```python
from build123d import *

# Parameters (mm, degrees)
SCHIZZO1_W                   = 27
SCHIZZO1_H                   = 20
SCHIZZO1_R                   = 1.4
ESTRUSIONE_ESTRUSIONE1_DEPTH = 2
RACCORDO1_R                  = 3
SCHIZZO2_R                   = 1.75
ESTRUSIONE_ESTRUSIONE2_DEPTH = 2.4
SCHIZZO3_R                   = 3
SCHIZZO3_R_2                 = 1.4
ESTRUSIONE_ESTRUSIONE3_DEPTH = 3


with BuildPart() as part:
    # Schizzo1 → Estrusione-Estrusione1 (new body)
    with BuildSketch(Plane.XY):
        Rectangle(SCHIZZO1_W, SCHIZZO1_H)
        with Locations((-10.5, 7)):
            Circle(SCHIZZO1_R, mode=Mode.SUBTRACT)
        with Locations((-10.5, -5.3)):
            Circle(SCHIZZO1_R, mode=Mode.SUBTRACT)
        with Locations((10.5, -5.3)):
            Circle(SCHIZZO1_R, mode=Mode.SUBTRACT)
        with Locations((10.5, 7)):
            Circle(SCHIZZO1_R, mode=Mode.SUBTRACT)
    extrude(amount=ESTRUSIONE_ESTRUSIONE1_DEPTH)

    # Raccordo1
    raccordo1_edges = [part.edges().sort_by_distance(p)[0] for p in [
        (-13.5, 10, 1),
        (13.5, 10, 1),
    ]]
    fillet(raccordo1_edges, radius=RACCORDO1_R)

    # Schizzo2 → Estrusione-Estrusione2 (add)
    with BuildSketch(Plane(origin=(13.5, 0, 0), x_dir=(0, 0, -1), z_dir=(1, 0, 0))):
        with BuildLine():
            Line((0, -10), (0, -14))
            ThreePointArc((0, -14), (-4.631989498, -17.094996434), (-5.718807717, -11.631192283))
            Line((-5.718807717, -11.631192283), (-2, -7.912384566))
            Line((-2, -7.912384566), (-2, -10))
            Line((-2, -10), (0, -10))
        make_face()
        with Locations((-3.35, -14)):
            Circle(SCHIZZO2_R, mode=Mode.SUBTRACT)
    estrusione_estrusione2 = extrude(amount=-ESTRUSIONE_ESTRUSIONE2_DEPTH)

    # Specchia1: Estrusione-Estrusione2 across plane
    add(estrusione_estrusione2.mirror(Plane(origin=(0, 0, 0), x_dir=(0, 0, 1), z_dir=(1, 0, 0))))

    # Schizzo3 → Estrusione-Estrusione3 (add)
    # profile 1 of 4: a face of its own
    with BuildSketch(Plane.XY.offset(2)):
        with Locations(Location((-10.5, 7, 0), (0, 0, 180))):
            Circle(SCHIZZO3_R)
        with Locations((-10.5, 7)):
            Circle(SCHIZZO3_R_2, mode=Mode.SUBTRACT)
    # profile 2 of 4: a face of its own
    with BuildSketch(Plane.XY.offset(2)):
        with Locations(Location((-10.5, -5.3, 0), (0, 0, 180))):
            Circle(SCHIZZO3_R)
        with Locations((-10.5, -5.3)):
            Circle(SCHIZZO3_R_2, mode=Mode.SUBTRACT)
    # profile 3 of 4: a face of its own
    with BuildSketch(Plane.XY.offset(2)):
        with Locations((10.5, -5.3)):
            Circle(SCHIZZO3_R)
        with Locations((10.5, -5.3)):
            Circle(SCHIZZO3_R_2, mode=Mode.SUBTRACT)
    # profile 4 of 4: a face of its own
    with BuildSketch(Plane.XY.offset(2)):
        with Locations((10.5, 7)):
            Circle(SCHIZZO3_R)
        with Locations((10.5, 7)):
            Circle(SCHIZZO3_R_2, mode=Mode.SUBTRACT)
    extrude(amount=ESTRUSIONE_ESTRUSIONE3_DEPTH)


solid = part.part
```
Model file for the job. Use its own axes, mm. A direction names the side the tool comes from. Coordinates: 2 decimals unless noted, no trailing zeros. Loops run counter-clockwise (first coordinate to the right, second up) from the corner with the lowest first, then second, coordinate; pieces in that order, holes last. Notation, with made-up numbers: M -8,-5 L 36,-5 A12 cw 36,0 Z; hole C 49.25,51 d3. An arc over 180 degrees is marked long. Use CSV: the item, a comma, the result in double quotes. Start each with the question number.
1. Band-saw the part on B-B, the plane x = -11.5. List the corners of the cut face in (y, z).
2. Flat gauge pins, fed straight in: pin 1 (3 mm diameter, centred on x = -4.5, y = 3.5, fed in from +Z); pin 2 (1.8 mm diameter, centred on x = -12, y = -6, fed in from +Z); pin 3 (3 mm diameter, centred on x = 3.5, z = 3, fed in from -Y); pin 4 (1.7 mm diameter, centred on x = 10.5, y = 7, fed in from -Z). Where does each tip first touch, or does it go through?
3. Band-saw the part on D-D, the plane x = -6.25. List the corners of the cut face in (y, z).
4. Band-saw the part on C-C, the plane y = -3.5. List the corners of the cut face in (x, z), then the cut area to 3 significant figures.
5. Band-saw the part on A-A, the plane z = 4.5. Give the number of separate pieces and of enclosed holes in the cut face, then the cut area to 3 significant figures.
6. Tool access for faces 1 (the cylindrical face through (-12.317, -12.265, 3.578)), 2 (the flat face through (0, -2, 0)), 3 (the flat face through (0, 0, 2)), 4 (the flat face through (-12, -6, 5)), 5 (the flat face through (-13.1, -7.4, 2)): list every direction of +Z, -Z, +X, -X, +Y, -Y with a clear straight run to the whole face (end or side of a thin tool).
7. Probe probe 1 along Y at (x, z) = (-10.5, 3.3); probe 2 along Y at (x, z) = (-10.5, 1.25); probe 3 along X at (y, z) = (-6.5, 1.5). List the from-to ranges inside material, lowest first. Write a range as [from, to].
8. Two-plate mould, pull along Y, no slides. Class faces 6 (the cylindrical face through (9.1, 7.06, 2.46)), 7 (the flat face through (-13.5, -7.7, 1.8)), 8 (the cylindrical face through (-12.317, -17.129, 4.546)), 9 (the cylindrical face through (-9.85, -2.37, 3.48)): pulls with the +Y half, pulls with the -Y half, needs draft (parallel to the pull), parting line crosses it, or undercut.
Entries:
1,outline,"M -14,0 L -6.28,0 L -6.28,5 L -8.13,5 L -8.13,2.22 L -11.63,5.72 A3.35 ccw long Z; M -4.32,0 L 6.02,0 L 6.02,5 L 4.17,5 L 4.17,2 L -2.47,2 L -2.47,5 L -4.32,5 Z; M 7.98,0 L 9.83,0 L 9.83,5 L 7.98,5 Z; hole C -14,3.35 d3.5"
2,pin 1,"stops at z = 2"
2,pin 2,"stops at z = 5"
2,pin 3,"stops at y = -10"
2,pin 4,"passes through"
3,outline,"M -10,0 L 10,0 L 10,2 L -10,2 Z"
4,outline,"M -13.5,0 L 13.5,0 L 13.5,2 L 12.9,2 L 12.9,5 L 8.1,5 L 8.1,2 L -8.1,2 L -8.1,5 L -12.9,5 L -12.9,2 L -13.5,2 Z"
4,area,"82.8 mm2"
5,separate pieces,"8"
5,enclosed holes,"4"
5,area,"108 mm2"
6,face 1,"+X, -X"
6,face 2,"-Z, +X, -X, +Y, -Y"
6,face 3,"+Z"
6,face 4,"+Z, +X, -X, +Y"
6,face 5,"+Z, -X"
7,probe 1,"y = [-8.3, -6.7], [-3.9, -2.3], [4, 5.6], [8.4, 10]"
7,probe 2,"y = [-10, -6.7], [-3.9, 5.6], [8.4, 10]"
7,probe 3,"x = [-13.5, -11.22], [-9.78, 9.78], [11.22, 13.5]"
8,face 6,"undercut"
8,face 7,"needs draft"
8,face 8,"parting line crosses it"
8,face 9,"undercut"
